Part model, mm, in its own coordinate system. Give positions to 0.01 mm unless a question says otherwise; leave off trailing zeros. Order: outer loops, then holes, each group sorted by start corner. A loop starts at its lowest first (then second) coordinate and runs counter-clockwise, first axis right, second up. Notation, with made-up numbers: (29, 83.25) -> (47, 83.25) arc R34 cw to (47, 120.25) -> close; hole circle Ø8 at (63, 21). An arc over 180 degrees is marked (long way). Write item = value, one per line. Start each with the question number.
(1) Two-plate mould, pull along X, no slides. Class faces 1 (the flat face through (-87, 0, 19)), 2 (the cylindrical face through (190.314, 3.219, 42.704)): pulls with the +X half, pulls with the -X half, needs draft (parallel to the pull), parting line crosses it, or undercut.
(2) Saw through at A-A, the plane x = -102.5. List the corners of the cut face in (y, z), then the cut area to 3 significant figures.
(3) Saw through at B-B, the plane z = 53.5. List the corners of the cut face in (x, y).
(4) Saw through at D-D, the plane x = -344. List the corners of the cut face in (y, z), then the cut area to 3 significant figures.
(5) Saw through at C-C, the plane y = 4. List the corners of the cut face in (x, z).
(6) Probe line 1 along X through (y, z) = (1.5, 44); line 2 along X through (y, z) = (2.5, 161); line 3 along X through (y, z) = (0.75, 284). List the from-to ranges inside material, lowest first. Write a range as from..to.
from build123d import *

# Parameters (mm, degrees)
SKETCH1_W           = 609.6
SKETCH1_H           = 609.6
BOSS_EXTRUDE1_DEPTH = 6.35
SKETCH2_R           = 44.45
CUT_EXTRUDE1_DEPTH  = 101.6


with BuildPart() as part:
    # Sketch1 → Boss-Extrude1 (new body)
    with BuildSketch(Plane(origin=(0, 0, 0), x_dir=(1, 0, 0), z_dir=(0, 1, 0))):
        with Locations((-82.357575758, -23.090909091)):
            Rectangle(SKETCH1_W, SKETCH1_H)
    extrude(amount=BOSS_EXTRUDE1_DEPTH)

    # Sketch2 → Cut-Extrude1 (cut)
    with BuildSketch(Plane(origin=(0, 6.35, 0), x_dir=(1, 0, 0), z_dir=(0, 1, 0))):
        with Locations(Location((-82.357575758, -169.140909091, 0), (0, 0, 270))):
            Circle(SKETCH2_R)
        with Locations((-82.357575758, -315.190909091)):
            Circle(SKETCH2_R)
        with Locations(Location((-310.957575758, -48.490909091, 0), (0, 0, 270))):
            Circle(SKETCH2_R)
        with Locations(Location((146.242424242, -48.490909091, 0), (0, 0, 270))):
            Circle(SKETCH2_R)
    extrude(amount=-CUT_EXTRUDE1_DEPTH, mode=Mode.SUBTRACT)


solid = part.part
Results list:
q1.face_1 = needs draft
q1.face_2 = undercut
q2.outline = (0, -281.71) -> (6.35, -281.71) -> (6.35, 129.52) -> (0, 129.52) -> close; (0, 208.77) -> (6.35, 208.77) -> (6.35, 275.57) -> (0, 275.57) -> close
q2.area = 3,040 mm^2
q3.outline = (-387.16, 0) -> (-355.12, 0) -> (-355.12, 6.35) -> (-387.16, 6.35) -> close; (-266.79, 0) -> (102.08, 0) -> (102.08, 6.35) -> (-266.79, 6.35) -> close; (190.41, 0) -> (222.44, 0) -> (222.44, 6.35) -> (190.41, 6.35) -> close
q4.outline = (0, -281.71) -> (6.35, -281.71) -> (6.35, 18.76) -> (0, 18.76) -> close; (0, 78.22) -> (6.35, 78.22) -> (6.35, 327.89) -> (0, 327.89) -> close
q4.area = 3,490 mm^2
q5.outline = (-387.16, -281.71) -> (222.44, -281.71) -> (222.44, 327.89) -> (-39.76, 327.89) arc R44.45 cw (long way) to (-124.95, 327.89) -> (-387.16, 327.89) -> close; hole circle Ø88.9 at (-310.96, 48.49); hole circle Ø88.9 at (-82.36, 169.14); hole circle Ø88.9 at (146.24, 48.49)
q6.line_1 = -387.16..-355.18, -266.74..102.02, 190.46..222.44
q6.line_2 = -387.16..-126.06, -38.66..222.44
q6.line_3 = -387.16..-114.03, -50.69..222.44
